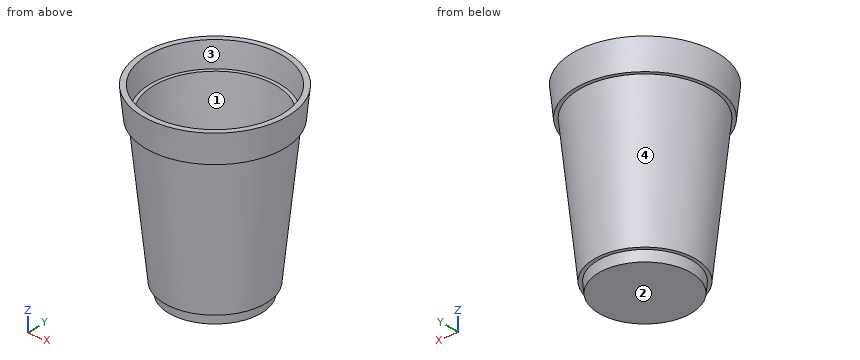
from build123d import *

# Parameters (mm, degrees)
THICKNESS_T = -3


with BuildPart() as part:
    # Sketch → Revolution (revolve)
    with BuildSketch(Plane.XZ):
        Polygon((0, 0), (-26.5, 0), (-27.091608, 5.970762), (-29.091608, 5.970762), (-37.723016, 88.093128), (-39.723016, 88.093128), (-41.5, 105), (0, 105), align=None)
    revolve(axis=Axis((0, 0, 0), (0, 0, 1)))

    # Thickness
    thickness_openings = [part.faces().sort_by_distance(p)[0] for p in [
        (0, 0, 105),
    ]]
    offset(amount=THICKNESS_T, openings=thickness_openings, kind=Kind.INTERSECTION)


solid = part.part
Part model, mm, in its own coordinate system. Face numbers are marked on the shaded views. Round coordinates to 2 decimals unless told otherwise and drop trailing zeros. Write each loop counter-clockwise with the first axis right and the second up, starting at its lowest first coordinate (ties: lowest second). Pieces come first, ordered by that corner, then holes. Notation, with made-up numbers: M 55,21 L 113,21 A29 ccw 113,43 Z; hole C 89,16 d3. An arc over 180 degrees is marked long. Return JSON: item names as keys, results as strings. Group by question number.
(1) Saw through at A-A on x = 0. Write the cut outline in (y, z).
(2) Drill centre lines: probe 1 along Z at (x, y) = (10, 12); probe 2 along X at (y, z) = (-19, 56); probe 3 along X at (y, z) = (-15.5, 48). Where is each one in solid material? Low to high.
(3) Saw through at C-C on z = 76. Write the cut outline in (x, y).
(4) Saw through at D-D on z = 35. Write the cut outline in (x, y).
(5) Pin check, flat tips, straight feed: pin 1 Ø4 at (x, z) = (-3, 30) entering from -Y; pin 2 Ø5 at (x, y) = (-0.5, -18.5) entering from +Z; pin 3 Ø6 at (y, z) = (5.5, 22.5) entering from -X. Stop position of each tip, or through.
(6) Two-plate mould, pull along Y, no slides. Class the marked faces 1, 2, 3 and 4: +Y half, -Y half, draft (parallel to the pull), parting line (faces both ways), or undercut.
Returned:
{
 "1": {"outline": "M -41.5,105 L -39.72,88.09 L -37.72,88.09 L -29.09,5.97 L -27.09,5.97 L -26.5,0 L 26.5,0 L 27.09,5.97 L 29.09,5.97 L 37.72,88.09 L 39.72,88.09 L 41.5,105 L 38.48,105 L 37.02,91.09 L 35.02,91.09 L 26.39,8.97 L 24.37,8.97 L 23.78,3 L -23.78,3 L -24.37,8.97 L -26.39,8.97 L -35.02,91.09 L -37.02,91.09 L -38.48,105 Z"},
 "2": {"probe 1": "0 to 3", "probe 2": "-28.62 to -24.92, 24.92 to 28.62", "probe 3": "-29.71 to -26.26, 26.26 to 29.71"},
 "3": {"outline": "C 0,0 d72.9; hole C 0,0 d66.87"},
 "4": {"outline": "C 0,0 d64.29; hole C 0,0 d58.25"},
 "5": {"pin 1": "y = -31.74", "pin 2": "z = 3", "pin 3": "x = -30.87"},
 "6": {"face 1": "undercut", "face 2": "draft", "face 3": "undercut", "face 4": "parting line"}
}
